Verification items for the finished model (mm, model axes). Face numbers are marked on the shaded views. A direction names the side the tool comes from. Round coordinates to 2 decimals unless told otherwise and drop trailing zeros. Write each question's results on one line, items separated by ' | '.
from build123d import *

# Parameters (mm, degrees)
F5_DEPTH = 50


with BuildPart() as f5:
    # F4 (on 3pt) → F5 (new body)
    with BuildSketch(Plane(origin=(-25, 0, 0), x_dir=(0, -1, 0), z_dir=(-1, 0, 0))):
        with BuildLine():
            ThreePointArc((-1.0401698304, 43.2797124187), (6.8786729535, 39.066003665), (10.8033382098, 31))
            Line((10.8033382098, 31), (22.0580684066, 31))
            Line((22.0580684066, 31), (22.0580684066, 39.2068698107))
            Line((22.0580684066, 39.2068698107), (-1.0401698304, 43.2797124187))
        make_face()
        with BuildLine():
            Line((8.7808942727, 31), (10.8033382098, 31))
            ThreePointArc((10.8033382098, 31), (6.8786729535, 39.066003665), (-1.0401698304, 43.2797124187))
            ThreePointArc((-1.0401698304, 43.2797124187), (-12.878488747, 40.1076444252), (-18.0580684066, 29))
            Line((-18.0580684066, 29), (-16.0580684066, 29))
            ThreePointArc((-16.0580684066, 29), (-4.5613047968, 41.4596756276), (8.7808942727, 31))
        make_face()
    extrude(amount=-F5_DEPTH)

    # F6: sweep along a path in F6_path
    with BuildLine(Plane(origin=(25, 18.0580684066, 29), x_dir=(0, 1, 0), z_dir=(-1, 0, 0))) as f6_path:
        ThreePointArc((0, 0), (-5.1795796595, -11.1076444252), (-17.0178985762, -14.2797124187))
        Line((-17.0178985762, -14.2797124187), (-40.1161368131, -10.2068698107))
    # F2 (on offset) → F6 (sweep)
    with BuildSketch(Plane.XY.offset(29)):
        with BuildLine():
            ThreePointArc((25, 18.0580684066), (12.6589889012, 21.0517490389), (0, 22.0580684066))
            ThreePointArc((0, 22.0580684066), (-12.6589889012, 21.0517490389), (-25, 18.0580684066))
            Line((-25, 18.0580684066), (25, 18.0580684066))
        make_face()
    sweep(path=f6_path.line)


solid = f5.part
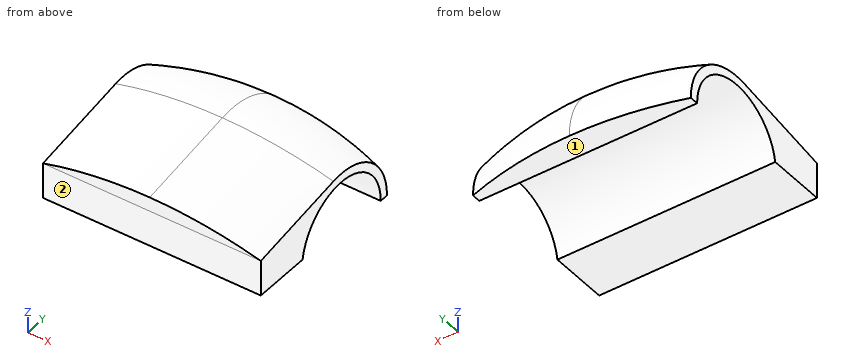
1) Material ranges on line 1 (Y direction, x = 13, z = 34.5); line 2 (Y direction, x = 8, z = 33.5); line 3 (Z direction, x = -5.5, y = 20.5), recorded low to high. Write a range as [from, to].
Calculated:
line 1: y = [-22.06, -7.67], [14.78, 20.11] | line 2: y = [-22.06, -8.1], [15.22, 21.09] | line 3: z = [29, 35.95]
2) Depth check by flat-ended pin: P1, Ø2.5, axis at x = -8.5, z = 36.5, coming from the -Y side; P2, Ø14.5, axis at x = 8.5, y = -15.5, coming from the -Z side; P3, Ø1.5, axis at x = -6, y = -1.5, coming from the +Z side; P4, Ø8, axis at x = -1.5, z = 39.5, coming from the -Y side. Enter the tip coordinate at first touch or a pass-through.
Calculated:
P1: stops at y = -22.06 | P2: stops at z = 31 | P3: stops at z = 46.81 | P4: stops at y = -22.75
3) Access from +Z, -Z, +X, -X, +Y, -Y to the whole of each face (thin tool, end or side, straight path). Record for the marked faces 1 and 2.
Calculated:
face 1: -Z, +X, -X, +Y, -Y | face 2: -Z, +X, -X, -Y
